from build123d import *

# Parameters (mm, degrees)
F0_W     = 151.8304795027
F0_H     = 151.7131924629
F1_DEPTH = 127
F2_T     = -7.62
F3_W     = 6.8829804659
F3_H     = 151.7131924629
F4_DEPTH = 76.2
F5_W     = 17.6434051245
F5_H     = 27.9590406418
F6_DEPTH = 0.254
F7_W     = 17.6434051245
F7_H     = 15.647560358
F8_DEPTH = 0.254


with BuildPart() as f1:
    # F0 (on Top) → F1 (new body)
    with BuildSketch(Plane.XY):
        Rectangle(F0_W, F0_H)
    extrude(amount=F1_DEPTH)

    # F2
    f2_openings = [f1.faces().sort_by_distance(p)[0] for p in [
        (0, 0, 127),
    ]]
    offset(amount=F2_T, openings=f2_openings)

    # F3 (on face) → F4 (join)
    with BuildSketch(Plane.XY.offset(127)):
        with Locations((71.7989727855, 0)):
            Rectangle(F3_W, F3_H)
    extrude(amount=F4_DEPTH)

    # F5 (on face) → F6 (join)
    with BuildSketch(Plane(origin=(-75.9152397513, 0, 0), x_dir=(0, -1, 0), z_dir=(-1, 0, 0))):
        with Locations((0, 113.0204796791)):
            Rectangle(F5_W, F5_H)
    extrude(amount=F6_DEPTH)

    # F7 (on face) → F8 (join)
    with BuildSketch(Plane(origin=(-76.1692397513, 0, 0), x_dir=(0, -1, 0), z_dir=(-1, 0, 0))):
        with Locations((0, 113.0204796791)):
            Rectangle(F7_W, F7_H)
    extrude(amount=F8_DEPTH)


solid = f1.part
Check sheet for the modelled part. Datum: model origin and axes. Units: mm. A direction names the side the tool comes from. Give positions to 0.01 mm unless a question says otherwise; leave off trailing zeros. Loops run counter-clockwise (first coordinate to the right, second up) from the corner with the lowest first, then second, coordinate; pieces in that order, holes last. Notation, with made-up numbers: M 85,36 L 115,36 A32 cw 115,64 Z; hole C 88.25,-19 d6. An arc over 180 degrees is marked long. Answer as a JSON object with one key per item and string values. Group by question number.
Q1. Cross-section at A-A on z = 20. Record the cut outline in (x, y), then the cut area to 3 significant figures.
Q2. Cross-section at D-D on z = 177. Record the cut outline in (x, y), then the cut area to 3 significant figures.
Q3. Cross-section at B-B on x = 2.5. Record the cut outline in (y, z).
Q4. Material ranges on line 1 along X through (y, z) = (39, 80); line 2 along Y through (x, z) = (47, 111); line 3 along Z through (x, y) = (53.5, 24), recorded low to high. Write a range as [from, to].
Q5. Access from +Z, -Z, +X, -X, +Y, -Y to the whole of each face (thin tool, end or side, straight path). Record for faces 1 (the flat face through (-68.5, 0.4, 127)), 2 (the flat face through (75.24, -1, 165)), 3 (the flat face through (-1, -68.237, 66)).
Q6. Cross-section at C-C on y = 46. Record the cut outline in (x, z).
Q7. Release check for a two-part mould opening along X. For faces 4 (the flat face through (-76.169, 0, 102)), 5 (the flat face through (68.295, -1, 66)), 6 (the flat face through (75.915, -1, 63)), 7 (the flat face through (-1, 1, 7.62)) record: released by +X, released by -X, zero draft, split by the parting line, or undercut.
Q8. Go/stop test with flat-tipped pins: P1, Ø5, axis at y = -26.5, z = 46, coming from the -X side; P2, Ø6, axis at y = 2.5, z = 172.5, coming from the +X side; P3, Ø1.8, axis at y = 2, z = 124, coming from the -X side; P4, Ø0.6, axis at x = -76, z = 116, coming from the +Y side. Record where each tip stops, or that it passes through.
Evaluation:
{
 "1": {"outline": "M -75.92,-75.86 L 75.92,-75.86 L 75.92,75.86 L -75.92,75.86 Z; hole M -68.3,-68.24 L 68.3,-68.24 L 68.3,68.24 L -68.3,68.24 Z", "area": "4,390 mm2"},
 "2": {"outline": "M 68.36,-75.86 L 75.24,-75.86 L 75.24,75.86 L 68.36,75.86 Z", "area": "1,040 mm2"},
 "3": {"outline": "M -75.86,0 L 75.86,0 L 75.86,127 L 68.24,127 L 68.24,7.62 L -68.24,7.62 L -68.24,127 L -75.86,127 Z"},
 "4": {"line 1": "x = [-75.92, -68.3], [68.3, 75.92]", "line 2": "y = [-75.86, -68.24], [68.24, 75.86]", "line 3": "z = [0, 7.62]"},
 "5": {"face 1": "+Z, -X, +Y, -Y", "face 2": "+Z, +X, +Y, -Y", "face 3": "+Z"},
 "6": {"outline": "M -75.92,0 L 75.92,0 L 75.92,127 L 75.24,127 L 75.24,203.2 L 68.36,203.2 L 68.36,127 L 68.3,127 L 68.3,7.62 L -68.3,7.62 L -68.3,127 L -75.92,127 Z"},
 "7": {"face 4": "released by -X", "face 5": "undercut", "face 6": "released by +X", "face 7": "undercut"},
 "8": {"P1": "stops at x = -75.92", "P2": "stops at x = 75.24", "P3": "stops at x = -76.17", "P4": "stops at y = 75.86"}
}
